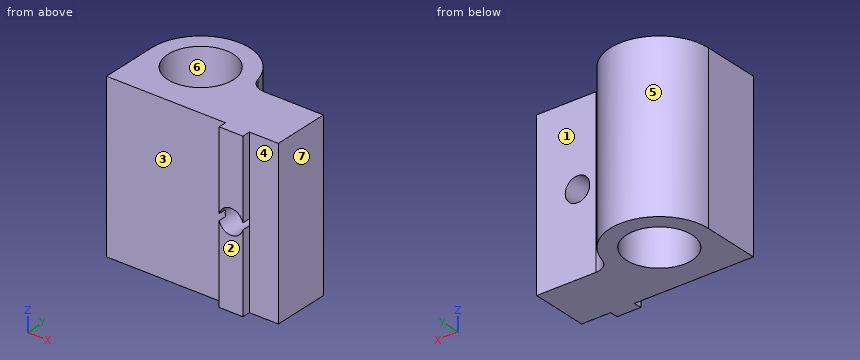
from build123d import *

# Parameters (mm, degrees)
SKETCH1_R                       = 4
MAIN_DEPTH                      = 10
SKETCH3_W                       = 2.9
SKETCH3_H                       = 20
MAKERBEAMRECTANGULARGUIDE_DEPTH = 1
SKETCH4_R                       = 1.5
MAKERBEAMFIXHOLE_DEPTH          = 9
FILLET1_R                       = 2


with BuildPart() as part:
    # Sketch1 → Main (new body, symmetric)
    with BuildSketch(Plane.XY):
        with BuildLine():
            Line((-6, 0), (-6, -7))
            Line((-6, -7), (15, -7))
            Line((15, -7), (15, 0))
            Line((15, 0), (6, 0))
            ThreePointArc((6, 0), (0, 6), (-6, 0))
        make_face()
        Circle(SKETCH1_R, mode=Mode.SUBTRACT)
    extrude(amount=MAIN_DEPTH, both=True)

    # Sketch3 → MakerBeamRectangularGuide (add)
    with BuildSketch(Plane(origin=(0, -7, 0), x_dir=(-1, 0, 0), z_dir=(0, -1, 0))):
        with Locations((-10, 0)):
            Rectangle(SKETCH3_W, SKETCH3_H)
    extrude(amount=MAKERBEAMRECTANGULARGUIDE_DEPTH)

    # Sketch4 → MakerBeamFixHole (cut, through all)
    with BuildSketch(Plane(origin=(0, 0, 0), x_dir=(1, 0, 0), z_dir=(0, 1, 0))):
        with Locations((10, 0)):
            Circle(SKETCH4_R)
    extrude(amount=-MAKERBEAMFIXHOLE_DEPTH, mode=Mode.SUBTRACT)

    # Fillet1
    fillet1_edges = [part.edges().sort_by_distance(p)[0] for p in [
        (6, 0, 0),
    ]]
    fillet(fillet1_edges, radius=FILLET1_R)


solid = part.part
Geometry check sheet. Reference: the model listing, model coordinates, mm. Face numbers are marked on the shaded views. A direction names the side the tool comes from. Give positions to 0.01 mm unless a question says otherwise; leave off trailing zeros. Write each loop counter-clockwise with the first axis right and the second up, starting at its lowest first coordinate (ties: lowest second). Pieces come first, ordered by that corner, then holes. Notation, with made-up numbers: M 79,-32 L 132,-32 A25 ccw 132,3 Z; hole C -12,-36 d5. An arc over 180 degrees is marked long. One line per question, with ' | ' between items.
1. Gauge pin test, flat ends, axial feed: pin 1 (8 mm diameter, centred on x = 3.5, z = -5.5, fed in from -Y); pin 2 (4 mm diameter, centred on x = 1, y = 2.5, fed in from -Z); pin 3 (0.8 mm diameter, centred on y = -7.5, z = 6, fed in from -X); pin 4 (1.5 mm diameter, centred on y = 4, z = 6.5, fed in from +X). Record the tip position at first contact, or that the pin passes through.
Ans:
pin 1: y = -7 | pin 2: z = -10 | pin 3: x = 8.55 | pin 4: x = 5.04
2. Mould release check, pull along X, two halves, no side actions. Record for the marked faces 5, 6 and 7: released by +X, released by -X, zero draft, split by the parting line, or undercut.
Ans:
face 5: split by the parting line | face 6: undercut | face 7: released by +X
3. Cross-section at C-C (y = -2.75). Enter the section's corners in (x, z), plus the area to 3 significant figures.
Ans:
outline: M -6,-10 L -2.9,-10 L -2.9,10 L -6,10 Z; M 2.9,-10 L 15,-10 L 15,10 L 2.9,10 Z; hole C 10,0 d3 | area: 297 mm2
4. Scan lines: line 1 along Z through (x, y) = (10, -2.25); line 2 along X through (y, z) = (-3, -0.25); line 3 along Y through (x, z) = (0, -2). Record each from-to range of solid material in increasing order. Write a range as from..to.
Ans:
line 1: -10..-1.5, 1.5..10 | line 2: -6..-2.65, 2.65..8.52, 11.48..15 | line 3: -7..-4, 4..6
5. Cross-section at D-D (z = -5.75). Enter the section's corners in (x, y), plus the area to 3 significant figures.
Ans:
outline: M -6,-7 L 8.55,-7 L 8.55,-8 L 11.45,-8 L 11.45,-7 L 15,-7 L 15,0 L 7.75,0 A2 cw 5.81,1.5 A6 ccw -6,0 Z; hole C 0,0 d8 | area: 157 mm2
6. Set-up check for the marked faces 1, 2, 3 and 4: record each of +Z, -Z, +X, -X, +Y, -Y from which the full face is reachable in a straight line by a thin tool's end or side.
Ans:
face 1: +Z, -Z, +X, +Y | face 2: +Z, -Z, +X, -X, -Y | face 3: +Z, -Z, -X, -Y | face 4: +Z, -Z, +X, -Y
7. Cross-section at B-B (x = 10). Enter the section's corners in (y, z).
Ans:
outline: M -8,-10 L 0,-10 L 0,-1.5 L -8,-1.5 Z; M -8,1.5 L 0,1.5 L 0,10 L -8,10 Z
8. Cross-section at A-A (z = 0). Enter the section's corners in (x, y).
Ans:
outline: M -6,-7 L 8.5,-7 L 8.5,0 L 7.75,0 A2 cw 5.81,1.5 A6 ccw -6,0 Z; M 11.5,-7 L 15,-7 L 15,0 L 11.5,0 Z; hole C 0,0 d8
